Verification items for the finished model (mm, model axes). A direction names the side the tool comes from. Give positions to 0.01 mm unless a question says otherwise; leave off trailing zeros. Loops run counter-clockwise (first coordinate to the right, second up) from the corner with the lowest first, then second, coordinate; pieces in that order, holes last. Notation, with made-up numbers: M 82.5,1 L 109.5,1 A32 cw 109.5,37 Z; hole C 87.25,73 d10. An arc over 180 degrees is marked long. Put each result on its own line as item: value. Start each with the question number.
from build123d import *

# Parameters (mm, degrees)
ESQUISSE1_W             = 96.6
ESQUISSE1_H             = 32
BOSS_EXTRU_1_DEPTH      = 1
ESQUISSE6_R             = 3.5
BOSS_EXTRU_2_DEPTH      = 33
ESQUISSE7_R             = 3
ESQUISSE7_R_2           = 5
ENL_V_MAT_EXTRU_1_DEPTH = 63.350617772


with BuildPart() as part:
    # Esquisse1 → Boss.-Extru.1 (new body)
    with BuildSketch(Plane.XY):
        with Locations((0.671156739, 2.259938231)):
            Rectangle(ESQUISSE1_W, ESQUISSE1_H)
    extrude(amount=BOSS_EXTRU_1_DEPTH)

    # Esquisse6 → Boss.-Extru.2 (add)
    with BuildSketch(Plane.XY.offset(1)):
        with Locations((-31.628843261, 2.259938231)):
            Circle(ESQUISSE6_R)
        with Locations((32.971156739, 2.259938231)):
            Circle(ESQUISSE6_R)
    extrude(amount=BOSS_EXTRU_2_DEPTH)

    # Esquisse7 → Enlèv. mat.-Extru.1 (cut, through all)
    with BuildSketch(Plane.XY.offset(34)):
        with Locations((-31.628843261, 2.259938231)):
            Circle(ESQUISSE7_R)
        with Locations((32.971156739, 2.259938231)):
            Circle(ESQUISSE7_R)
        with Locations((0.671156739, 2.259938231)):
            Circle(ESQUISSE7_R_2)
    extrude(amount=-ENL_V_MAT_EXTRU_1_DEPTH, mode=Mode.SUBTRACT)


solid = part.part
Q1. Set-up check for faces 4 (the face through (-34.626, 2.392, 17.238)), 5 (the face through (-28.396, 0.919, 17.269)): record each of +Z, -Z, +X, -X, +Y, -Y from which the full face is reachable in a straight line by a thin tool's end or side.
Q2. Cross-section at C-C, the plane y = -11. Record the boundary of the cut face in (x, z), then the cut area to 3 significant figures.
Q3. Release check for a two-part mould opening along Y. For faces 1 (the face through (0, 10, 1)), 2 (the face through (29.475, 2.414, 17.269)), 3 (the face through (29.974, 2.392, 17.238)) record: pulls with the +Y half, pulls with the -Y half, needs draft (parallel to the pull), parting line crosses it, or undercut.
Q4. Cross-section at A-A, the plane x = 34. Record the boundary of the cut face in (y, z), then the cut area to 3 significant figures.
Q5. Scan lines: L1, parallel to X at y = 5, z = 11.5; L2, parallel to X at y = 0.5, z = 13; L3, parallel to Z at x = -5, y = -3. Record each from-to range of solid material in increasing order.
Q6. Cross-section at B-B, the plane z = 24. Record the boundary of the cut face in (x, y).
Q7. Go/stop test with flat-tipped pins: pin 1 (13 mm diameter, centred on x = 0.67, y = 2.26, fed in from +Z); pin 2 (5 mm diameter, centred on x = 38, z = 16, fed in from +Y); pin 3 (3 mm diameter, centred on y = -1.5, z = 23.5, fed in from +X). Record where each tip stops, or that it passes through.
Ans:
1. face 4: +Z, -Z
1. face 5: +Z
2. outline: M -47.63,0 L 48.97,0 L 48.97,1 L -47.63,1 Z
2. area: 96.6 mm^2
3. face 1: needs draft
3. face 2: parting line crosses it
3. face 3: undercut
4. outline: M -13.74,0 L -0.56,0 L -0.56,34 L -1.09,34 L -1.09,1 L -13.74,1 Z; M 5.08,0 L 18.26,0 L 18.26,1 L 5.61,1 L 5.61,34 L 5.08,34 Z
4. area: 61.2 mm^2
5. L1: x = -33.81 to -32.85, -30.41 to -29.45, 30.79 to 31.75, 34.19 to 35.15
5. L2: x = -34.65 to -34.06, -29.2 to -28.6, 29.95 to 30.54, 35.4 to 36
5. L3: z = 0 to 1
6. outline: C -31.63,2.26 d7; C 32.97,2.26 d7; hole C -31.63,2.26 d6; hole C 32.97,2.26 d6
7. pin 1: stops at z = 1
7. pin 2: stops at y = 4.68
7. pin 3: stops at x = 35.64
